Work out the finished part from the listing and answer in its coordinate system (mm). A direction names the side the tool comes from. Round coordinates to 2 decimals unless told otherwise and drop trailing zeros. Write each loop counter-clockwise with the first axis right and the second up, starting at its lowest first coordinate (ties: lowest second). Pieces come first, ordered by that corner, then holes. Notation, with made-up numbers: (-13, -35.75) -> (15, -35.75) arc R7 ccw to (15, -24.75) -> close; hole circle Ø7 at (-31, -6.5). An arc over 180 degrees is marked (long way). Answer as a JSON object with one key per item and string values. Group by question number.
from build123d import *

# Parameters (mm, degrees)
F0_R            = 25.625
F1_DEPTH        = 0.5
F2_R            = 24.5
F3_DEPTH        = 30
F4_R            = 19.2
F5_DEPTH        = 30.501
F7_DEPTH        = 30
F7_COPIES_COUNT = 10


# Not quite as in the source:
# - a pattern or mirror of a feature is missing from the dataset's text; its kind, count and spacing are read off the source's solid


with BuildPart() as f1:
    # F0 (on Top) → F1 (new body)
    with BuildSketch(Plane.XY):
        Circle(F0_R)
    extrude(amount=F1_DEPTH)

    # F2 (on face) → F3 (join)
    with BuildSketch(Plane.XY.offset(0.5)):
        Circle(F2_R)
    extrude(amount=F3_DEPTH)

    # F4 (on face) → F5 (cut, through all)
    with BuildSketch(Plane.XY.offset(30.5)):
        Circle(F4_R)
    extrude(amount=-F5_DEPTH, mode=Mode.SUBTRACT)

    # F6 (on face) → F7 (cut, through all)
    with BuildSketch(Plane.XY.offset(30.5)):
        with BuildLine():
            Line((4.969325666, 18.5457758648), (6.341066605, 23.6651827441))
            ThreePointArc((6.341066605, 23.6651827441), (3.1978917094, 24.2903991037), (0, 24.5))
            Line((0, 24.5), (0, 19.2))
            ThreePointArc((0, 19.2), (2.5061028906, 19.0357413384), (4.969325666, 18.5457758648))
        make_face()
    f7 = extrude(amount=-F7_DEPTH, mode=Mode.SUBTRACT)

    # F7_copies: F7 ×10 about axis
    f7_copies_axis = Axis((0, 0, 0), (0, 0, 1))
    for i in range(1, F7_COPIES_COUNT):
        add(f7.rotate(f7_copies_axis, i * 360 / F7_COPIES_COUNT), mode=Mode.SUBTRACT)


solid = f1.part
1) Each of these flat-tipped pins is pushed along its axis until it touches: P1, Ø1, axis at y = 16, z = 3.5, coming from the -X side; P2, Ø10, axis at x = 19.5, z = 14.5, coming from the -Y side; P3, Ø10, axis at y = -20, z = 11.5, coming from the +X side. Where does it stop, or does it pass through?
2) A cutting plane is placed at D-D on y = -8.5. Determine the outline of the cut face in (x, z), plus the area to 3 significant figures.
3) A cutting plane is placed at C-C on x = -10.5. Determine the outline of the cut face in (y, z) (3 decimals), plus the area to 3 significant figures.
4) A tool of negligible diameter and unlimited length cuts with its end or side. For faces 1 (the face through (10.6, 22.09, 15.29)), 2 (the face through (-16.952, -13.727, 15.71)), 3 (the face through (-20.816, -6.763, 15.71)), 4 (the face through (-21.56, -11.64, 15.29)), 5 (the face through (-12.865, 17.707, 15.71)), from which of +Z, -Z, +X, -X, +Y, -Y can it reach the whole face along a straight path? Write none if from no direction.
5) For a pull along Y with two mould halves and no side action, classify faces 6 (the face through (20.816, -6.763, 15.71)), 7 (the face through (12.865, -17.707, 15.71)), 8 (the face through (-17.73, 16.91, 15.29)) as released by +Y, released by -Y, zero draft, split by the parting line, or undercut.
6) A cutting plane is placed at A-A on y = 0. Determine the outline of the cut face in (x, z) (3 decimals).
7) Straight lines are drawn through the part: L1, parallel to X at y = 0, z = 19.5; L2, parallel to Z at x = -13.5, y = -17; L3, parallel to Y at x = -15.5, z = 14. For each, find the intervals that lie inside material, in ascending order.
8) A cutting plane is placed at B-B on z = 25.5. State how many separate pieces and enclosed holes the cut face has, plus the area to 3 significant figures.
Established:
{
 "1": {"P1": "stops at x = -18.97", "P2": "stops at y = -19.75", "P3": "stops at x = 19.37"},
 "2": {"outline": "(-24.17, 0) -> (-17.22, 0) -> (-17.22, 30.5) -> (-22.98, 30.5) -> (-22.98, 0.5) -> (-24.17, 0.5) -> close; (17.22, 0) -> (24.17, 0) -> (24.17, 0.5) -> (17.22, 0.5) -> close", "area": "180 mm²"},
 "3": {"outline": "(-23.375, 0) -> (-16.075, 0) -> (-16.075, 30.5) -> (-22.136, 30.5) -> (-22.136, 0.5) -> (-23.375, 0.5) -> close; (16.075, 0) -> (23.375, 0) -> (23.375, 0.5) -> (16.075, 0.5) -> close", "area": "189 mm²"},
 "4": {"face 1": "+Z, +X, +Y", "face 2": "+Z, -Y", "face 3": "+Z, -X", "face 4": "+Z, -X, -Y", "face 5": "+Z, +Y"},
 "5": {"face 6": "undercut", "face 7": "released by -Y", "face 8": "released by +Y"},
 "6": {"outline": "(-25.625, 0) -> (-19.2, 0) -> (-19.2, 30.5) -> (-24.5, 30.5) -> (-24.5, 0.5) -> (-25.625, 0.5) -> close; (19.2, 0) -> (25.625, 0) -> (25.625, 0.5) -> (24.5, 0.5) -> (24.5, 30.5) -> (19.2, 30.5) -> close"},
 "7": {"L1": "x = -24.5 to -19.2, 19.2 to 24.5", "L2": "z = 0 to 0.5", "L3": "y = -12.55 to -11.33, 11.33 to 18.97"},
 "8": {"separate pieces": "10", "enclosed holes": "0", "area": "424 mm²"}
}
